```python
from build123d import *

# Parameters (mm, degrees)
SKETCH2_R                   = 88.9
BOSS_EXTRUDE1_DEPTH         = 3.175
SKETCH4_W                   = 15
SKETCH4_H                   = 17
SKETCH4_W_2                 = 21.412198496
SKETCH4_H_2                 = 63.5
CUT_EXTRUDE2_DEPTH          = 126.763669734
CIRPATTERN1_COUNT           = 3
CUT_EXTRUDE3_DEPTH          = 126.763669734
SKETCH8_R                   = 94.275983059
SKETCH8_R_2                 = 86.655983059
CUT_EXTRUDE_THIN1_DEPTH     = 126.763669734
SKETCH9_R                   = 3.175
CUT_EXTRUDE4_DEPTH          = 123.591188203
CIRPATTERN2_COUNT           = 3
SKETCH11_R                  = 1.5875
CUT_EXTRUDE6_DEPTH          = 123.591188203
CIRPATTERN3_COUNT           = 2
CIRPATTERN3_ANGLE           = 120
CIRPATTERN3_COPY_1_SKETCH_R = 1.5875
CIRPATTERN3_COPY_1_DEPTH    = 123.591188203
SKETCH12_R                  = 1.5875
CUT_EXTRUDE7_DEPTH          = 123.591188203
CIRPATTERN4_COUNT           = 2
CIRPATTERN4_ANGLE           = 120
CUT_EXTRUDE8_DEPTH          = 150
FILLET1_R                   = 22.86


with BuildPart() as part:
    # Sketch2 → Boss-Extrude1 (new body)
    with BuildSketch(Plane(origin=(0, 0, 0), x_dir=(1, 0, 0), z_dir=(0, 1, 0))):
        with Locations(Location((0, 0, 0), (0, 0, 270))):
            Circle(SKETCH2_R)
    extrude(amount=BOSS_EXTRUDE1_DEPTH)

    # Sketch4 → Cut-Extrude2 (cut, through all)
    with BuildSketch(Plane(origin=(0, 3.175, 0), x_dir=(1, 0, 0), z_dir=(0, 1, 0))):
        Polygon((23.51, 15.5), (16.51, 15.5), (16.51, -15.5), (23.51, -15.5), (23.51, -8.5), (23.51, 8.5), align=None)
        with Locations((73.13, 0)):
            Rectangle(SKETCH4_W, SKETCH4_H)
        with Locations((31.01, 0)):
            Rectangle(SKETCH4_W, SKETCH4_H)
        with Locations((91.336099248, 0)):
            Rectangle(SKETCH4_W_2, SKETCH4_H_2)
    cut_extrude2 = extrude(amount=-CUT_EXTRUDE2_DEPTH, mode=Mode.SUBTRACT)

    # CirPattern1: Cut-Extrude2 ×3 about axis
    cirpattern1_axis = Axis((0, 0, 0), (0, 1, 0))
    for i in range(1, CIRPATTERN1_COUNT):
        add(cut_extrude2.rotate(cirpattern1_axis, i * 360 / CIRPATTERN1_COUNT), mode=Mode.SUBTRACT)

    # Sketch6 → Cut-Extrude3 (cut, through all)
    with BuildSketch(Plane(origin=(0, 3.175, 0), x_dir=(1, 0, 0), z_dir=(0, 1, 0))):
        Polygon((-21.678393759, -6.548079416), (-21.678393759, 6.548079416), (5.168393759, 22.048079416), (16.51, 15.5), (16.51, -15.5), (5.168393759, -22.048079416), align=None)
    extrude(amount=-CUT_EXTRUDE3_DEPTH, mode=Mode.SUBTRACT)

    # Sketch8 → Cut-Extrude-Thin1 (cut, through all)
    with BuildSketch(Plane(origin=(0, 3.175, 0), x_dir=(1, 0, 0), z_dir=(0, 1, 0))):
        Circle(SKETCH8_R)
        Circle(SKETCH8_R_2, mode=Mode.SUBTRACT)
    extrude(amount=-CUT_EXTRUDE_THIN1_DEPTH, mode=Mode.SUBTRACT)

    # Sketch9 → Cut-Extrude4 (cut, through all)
    with BuildSketch(Plane(origin=(0, 3.175, 0), x_dir=(1, 0, 0), z_dir=(0, 1, 0))):
        with Locations(Location((65.549718535, 24.13, 0), (0, 0, 270))):
            Circle(SKETCH9_R)
        with Locations(Location((65.549718535, -24.13, 0), (0, 0, 90))):
            Circle(SKETCH9_R)
    cut_extrude4 = extrude(amount=-CUT_EXTRUDE4_DEPTH, mode=Mode.SUBTRACT)

    # CirPattern2: Cut-Extrude4 ×3 about axis
    cirpattern2_axis = Axis((0, 0, 0), (0, 1, 0))
    for i in range(1, CIRPATTERN2_COUNT):
        add(cut_extrude4.rotate(cirpattern2_axis, i * 360 / CIRPATTERN2_COUNT), mode=Mode.SUBTRACT)

    # Sketch11 → Cut-Extrude6 (cut, through all)
    with BuildSketch(Plane(origin=(0, 3.175, 0), x_dir=(1, 0, 0), z_dir=(0, 1, 0))):
        with Locations(Location((-74.764393759, 36.83, 0), (0, 0, 270))):
            Circle(SKETCH11_R)
        with Locations(Location((-62.064393759, 36.83, 0), (0, 0, 270))):
            Circle(SKETCH11_R)
        with Locations(Location((-74.764393759, 24.13, 0), (0, 0, 270))):
            Circle(SKETCH11_R)
    cut_extrude6 = extrude(amount=-CUT_EXTRUDE6_DEPTH, mode=Mode.SUBTRACT)

    # Mirror1: Cut-Extrude6 across plane
    add(cut_extrude6.mirror(Plane.XY), mode=Mode.SUBTRACT)

    # CirPattern3: Cut-Extrude6 ×2 about axis
    cirpattern3_axis = Axis((0, 0, 0), (0, 1, 0))
    for i in range(1, CIRPATTERN3_COUNT):
        add(cut_extrude6.rotate(cirpattern3_axis, i * CIRPATTERN3_ANGLE / (CIRPATTERN3_COUNT - 1)), mode=Mode.SUBTRACT)

    # CirPattern3 copy 1 sketch → CirPattern3 copy 1 (cut, through all)
    with BuildSketch(Plane(origin=(0, 3.175, 0), x_dir=(-0.5000000000000044, 0, -0.866025403784436), z_dir=(0, 1, 0))):
        with Locations((-74.764393759, -36.83)):
            Circle(CIRPATTERN3_COPY_1_SKETCH_R)
        with Locations((-62.064393759, -36.83)):
            Circle(CIRPATTERN3_COPY_1_SKETCH_R)
        with Locations((-74.764393759, -24.13)):
            Circle(CIRPATTERN3_COPY_1_SKETCH_R)
    extrude(amount=-CIRPATTERN3_COPY_1_DEPTH, mode=Mode.SUBTRACT)

    # Sketch12 → Cut-Extrude7 (cut, through all)
    with BuildSketch(Plane(origin=(0, 3.175, 0), x_dir=(1, 0, 0), z_dir=(0, 1, 0))):
        with Locations(Location((-33.108393759, 0, 0), (0, 0, 270))):
            Circle(SKETCH12_R)
        with BuildLine():
            ThreePointArc((-25.488393759, 5.3975), (-27.075893759, 3.81), (-25.488393759, 2.2225))
            Line((-25.488393759, 2.2225), (-25.488393759, 5.3975))
        make_face()
        with BuildLine():
            Line((-25.488393759, 5.3975), (-25.488393759, 2.2225))
            ThreePointArc((-25.488393759, 2.2225), (-24.365861744, 2.687467985), (-23.900893759, 3.81))
            ThreePointArc((-23.900893759, 3.81), (-24.365861744, 4.932532015), (-25.488393759, 5.3975))
        make_face()
        with BuildLine():
            ThreePointArc((-25.488393759, -2.2225), (-27.075893759, -3.81), (-25.488393759, -5.3975))
            Line((-25.488393759, -5.3975), (-25.488393759, -2.2225))
        make_face()
        with BuildLine():
            Line((-25.488393759, -2.2225), (-25.488393759, -5.3975))
            ThreePointArc((-25.488393759, -5.3975), (-24.365861744, -4.932532015), (-23.900893759, -3.81))
            ThreePointArc((-23.900893759, -3.81), (-24.365861744, -2.687467985), (-25.488393759, -2.2225))
        make_face()
    cut_extrude7 = extrude(amount=-CUT_EXTRUDE7_DEPTH, mode=Mode.SUBTRACT)

    # CirPattern4: Cut-Extrude7 ×2 about axis
    cirpattern4_axis = Axis((0, 0, 0), (0, 1, 0))
    for i in range(1, CIRPATTERN4_COUNT):
        add(cut_extrude7.rotate(cirpattern4_axis, i * CIRPATTERN4_ANGLE / (CIRPATTERN4_COUNT - 1)), mode=Mode.SUBTRACT)

    # Sketch10 → Cut-Extrude8 (cut)
    with BuildSketch(Plane(origin=(0, 3.175, 0), x_dir=(1, 0, 0), z_dir=(0, 1, 0))):
        Polygon((49.845863359, 15.215567884), (75.245863359, 59.209658396), (13.654136641, 94.769658396), (-11.745863359, 50.775567884), align=None)
    extrude(amount=-CUT_EXTRUDE8_DEPTH, mode=Mode.SUBTRACT)

    # Fillet1
    fillet1_edges = [part.edges().sort_by_distance(p)[0] for p in [
        (49.845863359, 1.5875, -15.215567884),
        (-11.745863359, 1.5875, -50.775567884),
    ]]
    fillet(fillet1_edges, radius=FILLET1_R)


solid = part.part
```
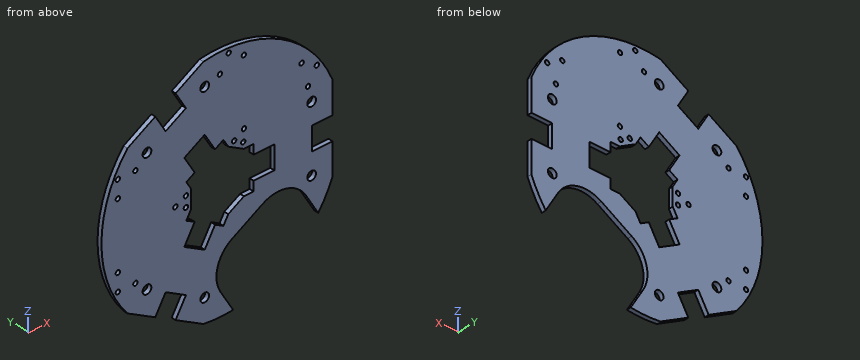
For this review, take the finished solid that the model builds, in its own axes (mm). Round coordinates to 2 decimals unless told otherwise and drop trailing zeros. One line per item, written item: value. Start each with the question number.
(1) Insertion check: pin 1 (1.6 mm diameter, centred on y = 2, z = 2, fed in from +X); pin 2 (2.5 mm diameter, centred on x = -62.06, z = 36.83, fed in from -Y); pin 3 (1.5 mm diameter, centred on x = 62, y = 0.5, fed in from +Z); pin 4 (1.6 mm diameter, centred on x = 69.5, y = 1.5, fed in from +Z). Each pin has a flat end and moves straight along its axis. Give the tip position at first contact, or say it passes through.
(2) We need section A-A (y = 0.65). Count the separate pieces of the cut face and the enclosed holes in it, and give its area (3 significant figures).
(3) Wall thickness on line 1 (X direction, y = 0.6, z = 0); line 2 (Z direction, x = 63, y = 0.6); line 3 (Z direction, x = -52, y = 2.65): over which ranges is each line inside the solid? List them lowest first.
Result:
1. pin 1: x = 65.63
1. pin 2: through
1. pin 3: z = 61.3
1. pin 4: z = 52.82
2. separate pieces: 1
2. enclosed holes: 25
2. area: 16,100 mm²
3. line 1: -86.66 to -34.7, -31.52 to -21.68, 38.51 to 65.63
3. line 2: -38 to -26.02, -22.24 to 22.24, 26.02 to 33.75, 36.92 to 59.5
3. line 3: -63.08 to -47.4, -42 to 42, 47.4 to 63.08
